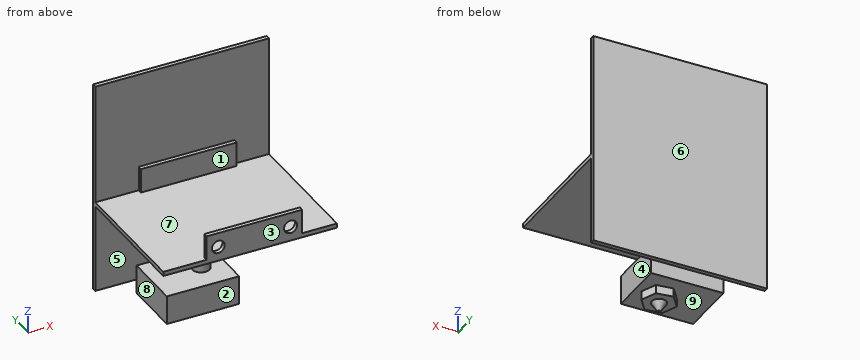
from build123d import *

# Parameters (mm, degrees)
F0_W      = 60
F0_H      = 74
F1_DEPTH  = 1.5
F2_W      = 33
F2_H      = 10
F3_DEPTH  = 1.5
F5_DEPTH  = 1.5
F6_W      = 33
F6_H      = 8.5
F6_H_2    = 1.5
F7_DEPTH  = 1.5
F8_R      = 2.2151606022
F8_R_2    = 2.2615912584
F9_DEPTH  = 2.5
F10_R     = 3
F11_DEPTH = 17
F12_W     = 25
F12_H     = 20
F12_R     = 3
F13_DEPTH = 10
F15_DEPTH = 3
F16_R     = 2.5
F17_DEPTH = 3
F18_SIZE2 = 2.99999
F18_SIZE  = 1.99999


# Not quite as in the source:
# - a fillet or chamfer is up to 0.001 mm smaller than in the source, because OpenCascade refuses the exact size


with BuildPart() as f1:
    # F0 (on Front) → F1 (new body)
    with BuildSketch(Plane.XZ):
        with Locations((-0.6031179801, 17)):
            Rectangle(F0_W, F0_H)
    extrude(amount=F1_DEPTH)

    # F2 (on face) → F3 (join)
    with BuildSketch(Plane.XZ.offset(1.5)):
        with Locations((0.8968820199, 15.5949131586)):
            Rectangle(F2_W, F2_H)
    extrude(amount=F3_DEPTH)

    # F4 (on face) → F5 (join)
    with BuildSketch(Plane(origin=(0, 0, 10.5949131586), x_dir=(1, 0, 0), z_dir=(0, 0, -1))):
        Polygon((-30.6031179801, 46.5), (-30.6031179801, 1.5), (-15.6031179801, 1.5), (-15.6031179801, 3), (17.3968820199, 3), (17.3968820199, 1.5), (29.3968820199, 1.5), (29.3968820199, 46.5), align=None)
    extrude(amount=-F5_DEPTH)

    # F6 (on face) → F7 (join)
    with BuildSketch(Plane.XZ.offset(46.5)):
        with Locations((0.8968820199, 16.3449131586)):
            Rectangle(F6_W, F6_H)
        with Locations((0.8968820199, 11.3449131586)):
            Rectangle(F6_W, F6_H_2)
    extrude(amount=-F7_DEPTH)

    # F8 (on face) → F9 (cut, symmetric)
    with BuildSketch(Plane.XZ.offset(46.5)):
        with Locations((-11.6031179801, 15.5949131586)):
            Circle(F8_R)
        with Locations((13.3968820199, 15.5949131586)):
            Circle(F8_R_2)
    extrude(amount=F9_DEPTH, both=True, mode=Mode.SUBTRACT)

    # F10 (on face) → F11 (join)
    with BuildSketch(Plane(origin=(0, 0, 10.5949131586), x_dir=(1, 0, 0), z_dir=(0, 0, -1))):
        with Locations((-5.6031179801, 23.5)):
            Circle(F10_R)
    extrude(amount=F11_DEPTH)

    # F12 (on face) → F13 (join)
    with BuildSketch(Plane(origin=(0, 0, -6.4050868414), x_dir=(1, 0, 0), z_dir=(0, 0, -1))):
        with Locations((-10.1031179801, 23.5)):
            Rectangle(F12_W, F12_H)
        with Locations((-5.6031179801, 23.5)):
            Circle(F12_R, mode=Mode.SUBTRACT)
        with Locations((-5.6031179801, 23.5)):
            Circle(F12_R)
    extrude(amount=F13_DEPTH)

    # F14 (on face) → F15 (join)
    with BuildSketch(Plane(origin=(0, 0, -16.4050868414), x_dir=(1, 0, 0), z_dir=(0, 0, -1))):
        Polygon((0.1261105875, 24.2136339076), (-3.3565287892, 28.8184744374), (-9.0857573568, 28.1048405298), (-11.3323465476, 22.7863660924), (-7.8497071709, 18.1815255626), (-2.1204786033, 18.8951594702), align=None)
    extrude(amount=F15_DEPTH)

    # F16 (on face) → F17 (join)
    with BuildSketch(Plane(origin=(0, 0, -19.4050868414), x_dir=(1, 0, 0), z_dir=(0, 0, -1))):
        with Locations((-5.6031179801, 23.5)):
            Circle(F16_R)
    extrude(amount=F17_DEPTH)

    # F18 (size 2 and 3 in the source; OpenCascade refuses exactly that, so slightly less here)
    f18_edges = [f1.edges().sort_by_distance(p)[0] for p in [
        (-8.103118, -23.5, -22.405087),
    ]]
    f18_side = f1.faces().sort_by_distance((-5.603118, -23.5, -22.405087))[0]
    chamfer(f18_edges, length=F18_SIZE, length2=F18_SIZE2, reference=f18_side)


solid = f1.part
Input: part model. Units: mm. Frame: model coordinates. Face numbers are marked on the shaded views. A direction names the side the tool comes from. Give positions to 0.01 mm unless a question says otherwise; leave off trailing zeros. Order: outer loops, then holes, each group sorted by start corner. A loop starts at its lowest first (then second) coordinate and runs counter-clockwise, first axis right, second up. Notation, with made-up numbers: (-35, -35) - (3, -35) arc R24 cw to (3, -17) - close; hole circle Ø8 at (66.5, 78). An arc over 180 degrees is marked (long way). Write each question's results on one line, items separated by ' | '.
Item 1: Material intervals for line 1 along Y through (x, z) = (-17.5, -15); line 2 along Z through (x, y) = (0.5, -19); line 3 along Z through (x, y) = (9.5, -40), sorted ascending.
A:
line 1: y = -33.5 to -13.5, -1.5 to 0 | line 2: z = -16.41 to -6.41, 10.59 to 12.09 | line 3: z = 10.59 to 12.09
Item 2: Draft query along Y for the marked faces 6, 7, 8 and 9. Return one class per face: released by +Y, released by -Y, zero draft, split by the parting line, or undercut.
A:
face 6: released by +Y | face 7: undercut | face 8: zero draft | face 9: undercut
Item 3: Section D-D (x = 12.5). Return loops of the section in (y, z), and give its area (3 significant figures).
A:
outline: (-46.5, 10.59) - (-1.5, 10.59) - (-1.5, -20) - (0, -20) - (0, 54) - (-1.5, 54) - (-1.5, 20.59) - (-3, 20.59) - (-3, 12.09) - (-45, 12.09) - (-45, 13.52) - (-46.5, 13.52) - close; (-46.5, 17.67) - (-45, 17.67) - (-45, 20.59) - (-46.5, 20.59) - close | area: 198 mm^2
Item 4: Section A-A (y = -32). Return loops of the section in (x, z).
A:
outline: (-30.6, 10.59) - (29.4, 10.59) - (29.4, 12.09) - (-30.6, 12.09) - close; (-22.6, -16.41) - (2.4, -16.41) - (2.4, -6.41) - (-22.6, -6.41) - close
Item 5: Access query for the marked faces 1, 2, 3, 4 and 5. Directions: +Z, -Z, +X, -X, +Y, -Y. A direction counts if a zero-diameter tool reaches every point of the face in a straight line with its end or side. Return the directions, or none.
A:
face 1: +Z, +X, -X | face 2: -Z, +X, -X, -Y | face 3: +Z, -Z, +X, -X, -Y | face 4: -Z, +X, -Y | face 5: -Z, +X, -X
Item 6: Section C-C (x = -26). Return loops of the section in (y, z).
A:
outline: (-46.5, 10.59) - (-1.5, 10.59) - (-1.5, -20) - (0, -20) - (0, 54) - (-1.5, 54) - (-1.5, 12.09) - (-46.5, 12.09) - close
Item 7: Contact query for flat-ended pins moving along their axis: pin 1 Ø1.6 at (x, y) = (-2.5, -45.5) entering from +Z; pin 2 Ø8.5 at (x, y) = (-7.5, -22) entering from -Z; pin 3 Ø1.2 at (y, z) = (-2.5, 18) entering from +X; pin 4 Ø3 at (x, y) = (-4.5, -6) entering from +Z. Output: stop coordinate, or through.
A:
pin 1: stops at z = 20.59 | pin 2: stops at z = -22.41 | pin 3: stops at x = 17.4 | pin 4: stops at z = 12.09
Item 8: Section B-B (z = -1). Return loops of the section in (x, y), and give its area (3 significant figures).
A:
outline: (-30.6, -1.5) - (29.4, -1.5) - (29.4, 0) - (-30.6, 0) - close; circle Ø6 at (-5.6, -23.5) | area: 118 mm^2
